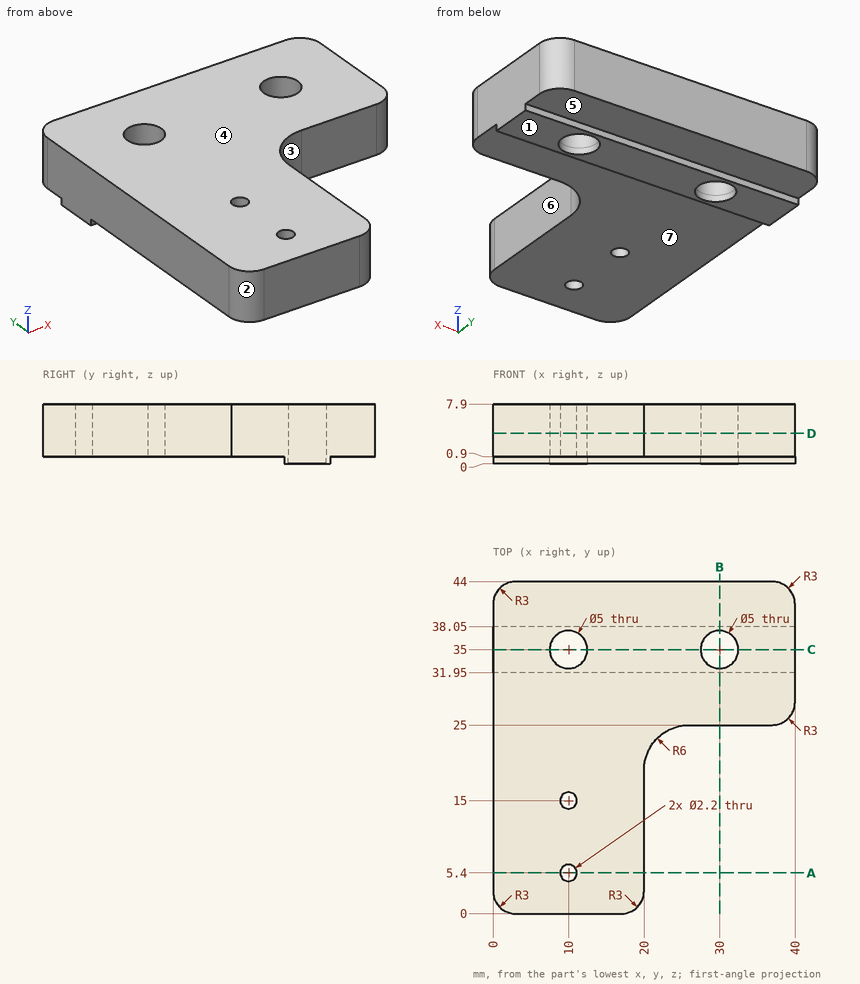
Can you work these out from the drawing? Everything is in mm from the part's minimum corner. A direction names the side the tool comes from. Coordinates: 2 decimals unless noted, no trailing zeros. Loops run counter-clockwise (first coordinate to the right, second up) from the corner with the lowest first, then second, coordinate; pieces in that order, holes last.
1. Imagine slicing it at C-C, the plane y = 35. Please give me the cut outline in (x, z).
2. Imagine slicing it at D-D, the plane z = 4. Please give me the cut outline in (x, y).
3. I need wall thicknesses on L1, parallel to Y at x = 10, z = 3.25; L2, parallel to Y at x = 9, z = 1.25; L3, parallel to X at y = 11.5, z = 7. Which ranges of each line are inside material? Lowest first, please.
4. For P1, Ø3, axis at x = 10, y = 5.4, coming from the -Z side; P2, Ø8, axis at x = 10, y = 35, coming from the -Z side; P3, Ø0.5, axis at x = 25, z = 0.5, coming from the -Y side; P4, Ø1.8, axis at x = 10, y = 15, coming from the -Z side, each with a flat end and sliding along its axis, tell me the tip position at first contact or that it passes through.
5. If we mould it in two halves opening along X, with no side actions, what happens to the marked faces 1, 2 and 3? For each: pulls with the +X half, pulls with the -X half, needs draft (parallel to the pull), parting line crosses it, or undercut.
6. For the marked faces 4, 5, 6 and 7, which set-ups out of +Z, -Z, +X, -X, +Y, -Y let a thin tool reach every point of the face, with its end or its side?
7. Imagine slicing it at B-B, the plane x = 30. Please give me the cut outline in (y, z), and give its area (3 significant figures).
8. Imagine slicing it at A-A, the plane y = 5.4. Please give me the cut outline in (x, z).
Taken from the geometry:
1. outline: (0, 0) - (7.5, 0) - (7.5, 7.9) - (0, 7.9) - close; (12.5, 0) - (27.5, 0) - (27.5, 7.9) - (12.5, 7.9) - close; (32.5, 0) - (40, 0) - (40, 7.9) - (32.5, 7.9) - close
2. outline: (0, 3) arc R3 ccw to (3, 0) - (17, 0) arc R3 ccw to (20, 3) - (20, 19) arc R6 cw to (26, 25) - (37, 25) arc R3 ccw to (40, 28) - (40, 41) arc R3 ccw to (37, 44) - (3, 44) arc R3 ccw to (0, 41) - close; hole circle Ø5 at (10, 35); hole circle Ø2.2 at (10, 5.4); hole circle Ø2.2 at (10, 15); hole circle Ø5 at (30, 35)
3. L1: y = 0 to 4.3, 6.5 to 13.9, 16.1 to 32.5, 37.5 to 44
3. L2: y = 0 to 4.94, 5.86 to 14.54, 15.46 to 32.71, 37.29 to 44
3. L3: x = 0 to 20
4. P1: stops at z = 0.9
4. P2: stops at z = 0
4. P3: stops at y = 31.95
4. P4: passes through
5. face 1: needs draft
5. face 2: pulls with the -X half
5. face 3: pulls with the +X half
6. face 4: +Z, +X, -X, +Y, -Y
6. face 5: -Z, +X, -X, +Y
6. face 6: +Z, -Z, +X, -Y
6. face 7: -Z, +X, -X, -Y
7. outline: (25, 0.9) - (31.95, 0.9) - (31.95, 0) - (32.5, 0) - (32.5, 7.9) - (25, 7.9) - close; (37.5, 0) - (38.05, 0) - (38.05, 0.9) - (44, 0.9) - (44, 7.9) - (37.5, 7.9) - close
7. area: 99.0 mm2
8. outline: (0, 0.9) - (8.9, 0.9) - (8.9, 7.9) - (0, 7.9) - close; (11.1, 0.9) - (20, 0.9) - (20, 7.9) - (11.1, 7.9) - close
